Geometry: final body of the model. Coordinates: model frame, mm. A direction names the side the tool comes from. Round coordinates to 2 decimals unless told otherwise and drop trailing zeros. Loops run counter-clockwise (first coordinate to the right, second up) from the corner with the lowest first, then second, coordinate; pieces in that order, holes last. Notation, with made-up numbers: (42, 42.5) - (95, 42.5) arc R10 cw to (95, 60.5) - close; hole circle Ø7 at (-2, 24). An arc over 180 degrees is marked (long way). Answer as a JSON object with one key per item and string values. Group by question number.
Item 1: Section C-C (y = -2). Return the cut outline in (x, z), plus the area to 3 significant figures.
Item 2: Reachability of faces 1 (the face through (0, 10, 0)), 2 (the face through (-5, 0, -2)) from +Z, -Z, +X, -X, +Y, -Y: full face, straight path, thin tool, end or side. Return the list, or none.
Item 3: First-contact query: pin 1 (12 mm diameter, centred on x = 0, y = -2, fed in from -Z); pin 2 (8 mm diameter, centred on x = 11.5, y = 6, fed in from -Z); pin 3 (12 mm diameter, centred on y = -3.5, z = -8.5, fed in from +X). Flat tips, straight axial feed; report the tip coordinate or a pass-through.
Item 4: Section D-D (y = 1). Return the cut outline in (x, z), plus the area to 3 significant figures.
Item 5: Line query: line 1 (Y direction, x = -1.5, z = -7); line 2 (Z direction, x = 8, y = 1.25); line 3 (Z direction, x = 13, y = 6.75). Output: solid intervals per line, ascending.
```python
from build123d import *

# Parameters (mm, degrees)
F0_R     = 15
F1_DEPTH = 10
F2_R     = 5
F3_DEPTH = 10
F4_R     = 5
F5_R     = 4.99999


# Not quite as in the source:
# - a fillet or chamfer is up to 0.001 mm smaller than in the source, because OpenCascade refuses the exact size


with BuildPart() as f1:
    # F0 (on Front) → F1 (new body)
    with BuildSketch(Plane.XZ):
        Circle(F0_R)
    extrude(amount=-F1_DEPTH)

    # F2 (on face) → F3 (join)
    with BuildSketch(Plane.XZ):
        Circle(F2_R)
    extrude(amount=F3_DEPTH)

    # F4
    f4_edges = [f1.edges().sort_by_distance(p)[0] for p in [
        (-15, 10, 0),
    ]]
    fillet(f4_edges, radius=F4_R)

    # F5 (radius 5 in the source; OpenCascade refuses exactly that, so slightly less here)
    f5_edges = [f1.edges().sort_by_distance(p)[0] for p in [
        (-15, 0, 0),
    ]]
    fillet(f5_edges, radius=F5_R)


solid = f1.part
```
Values:
{
 "1": {"outline": "circle Ø10 at (0, 0)", "area": "78.5 mm^2"},
 "2": {"face 1": "+Z, -Z, +X, -X, +Y", "face 2": "-Y"},
 "3": {"pin 1": "stops at z = -14.9", "pin 2": "stops at z = -12.95", "pin 3": "stops at x = 12.62"},
 "4": {"outline": "circle Ø26 at (0, 0)", "area": "531 mm^2"},
 "5": {"line 1": "y = 0 to 10", "line 2": "z = -10.63 to 10.63", "line 3": "z = -6.83 to 6.83"}
}
